from build123d import *

# Parameters (mm, degrees)
SKETCH1_R           = 20
BOSS_EXTRUDE1_DEPTH = 7
SKETCH2_R           = 8.5
CUT_EXTRUDE1_DEPTH  = 5
SKETCH3_R           = 4.5
CUT_EXTRUDE2_DEPTH  = 29.722813233
SKETCH4_R           = 1
CUT_EXTRUDE3_DEPTH  = 5
FILLET1_R           = 1


with BuildPart() as part:
    # Sketch1 → Boss-Extrude1 (new body)
    with BuildSketch(Plane(origin=(0, 0, 0), x_dir=(1, 0, 0), z_dir=(0, 1, 0))):
        with Locations(Location((0, 0, 0), (0, 0, 270))):
            Circle(SKETCH1_R)
    extrude(amount=BOSS_EXTRUDE1_DEPTH)

    # Sketch2 → Cut-Extrude1 (cut)
    with BuildSketch(Plane(origin=(0, 7, 0), x_dir=(1, 0, 0), z_dir=(0, 1, 0))):
        with Locations(Location((0, 0, 0), (0, 0, 270))):
            Circle(SKETCH2_R)
    extrude(amount=-CUT_EXTRUDE1_DEPTH, mode=Mode.SUBTRACT)

    # Sketch3 → Cut-Extrude2 (cut, through all)
    with BuildSketch(Plane(origin=(0, 2, 0), x_dir=(1, 0, 0), z_dir=(0, 1, 0))):
        with Locations(Location((0, 0, 0), (0, 0, 270))):
            Circle(SKETCH3_R)
    extrude(amount=-CUT_EXTRUDE2_DEPTH, mode=Mode.SUBTRACT)

    # Sketch4 → Cut-Extrude3 (cut)
    with BuildSketch(Plane(origin=(0, 7, 0), x_dir=(1, 0, 0), z_dir=(0, 1, 0))):
        with Locations(Location((0, 18, 0), (0, 0, 270))):
            Circle(SKETCH4_R)
        with Locations(Location((9, 15.588457268, 0), (0, 0, 270))):
            Circle(SKETCH4_R)
        with Locations(Location((15.588457268, 9, 0), (0, 0, 270))):
            Circle(SKETCH4_R)
        with Locations(Location((18, 0, 0), (0, 0, 270))):
            Circle(SKETCH4_R)
        with Locations(Location((15.588457268, -9, 0), (0, 0, 270))):
            Circle(SKETCH4_R)
        with Locations(Location((9, -15.588457268, 0), (0, 0, 270))):
            Circle(SKETCH4_R)
        with Locations(Location((0, -18, 0), (0, 0, 270))):
            Circle(SKETCH4_R)
        with Locations(Location((-9, -15.588457268, 0), (0, 0, 270))):
            Circle(SKETCH4_R)
        with Locations(Location((-15.588457268, -9, 0), (0, 0, 270))):
            Circle(SKETCH4_R)
        with Locations(Location((-18, 0, 0), (0, 0, 270))):
            Circle(SKETCH4_R)
        with Locations(Location((-15.588457268, 9, 0), (0, 0, 270))):
            Circle(SKETCH4_R)
        with Locations(Location((-9, 15.588457268, 0), (0, 0, 270))):
            Circle(SKETCH4_R)
    extrude(amount=-CUT_EXTRUDE3_DEPTH, mode=Mode.SUBTRACT)

    # Fillet1
    fillet1_edges = [part.edges().sort_by_distance(p)[0] for p in [
        (0, 0, -20),
    ]]
    fillet(fillet1_edges, radius=FILLET1_R)


solid = part.part
CAD build for the part. Positions are in the model's coordinates, mm. A direction names the side the tool comes from. Round coordinates to 2 decimals unless told otherwise and drop trailing zeros. Order: outer loops, then holes, each group sorted by start corner. A loop starts at its lowest first (then second) coordinate and runs counter-clockwise, first axis right, second up. Notation, with made-up numbers: M -30,-3.75 L -11,-3.75 A27 cw -11,35.25 Z; hole C 17,-30.75 d5. An arc over 180 degrees is marked long. Use one line per item in the form item = value.
Q1. Saw through at A-A on z = 0. Give the cut face in (x, y), then the cut area to 3 significant figures.
Recorded:
outline = M -20,1 A1 ccw -19,0 L -4.5,0 L -4.5,2 L -8.5,2 L -8.5,7 L -17,7 L -17,2 L -19,2 L -19,7 L -20,7 Z; M 4.5,0 L 19,0 A1 ccw 20,1 L 20,7 L 19,7 L 19,2 L 17,2 L 17,7 L 8.5,7 L 8.5,2 L 4.5,2 Z
area = 157 mm^2
Q2. Probe L1, parallel to X at y = 5.4, z = 0; L2, parallel to X at y = 6, z = 15; L3, parallel to X at y = 3.85, z = 9. List the from-to ranges inside material, lowest first.
Recorded:
L1 = -20 to -19, -17 to -8.5, 8.5 to 17, 19 to 20
L2 = -13.23 to -9.81, -8.19 to 8.19, 9.81 to 13.23
L3 = -17.86 to -16.59, -14.59 to 14.59, 16.59 to 17.86
Q3. Saw through at B-B on x = 0. Give the cut face in (y, z), then the cut area to 3 significant figures.
Recorded:
outline = M 0,-19 A1 ccw 1,-20 L 7,-20 L 7,-19 L 2,-19 L 2,-17 L 7,-17 L 7,-8.5 L 2,-8.5 L 2,-4.5 L 0,-4.5 Z; M 0,4.5 L 2,4.5 L 2,8.5 L 7,8.5 L 7,17 L 2,17 L 2,19 L 7,19 L 7,20 L 1,20 A1 ccw 0,19 Z
area = 157 mm^2
Q4. Flat gauge pins, fed straight in: P1, Ø4, axis at y = 2, z = 14, coming from the -X side; P2, Ø1, axis at x = 16, z = -9, coming from the +Y side; P3, Ø2, axis at x = 3.5, y = 3.5, coming from the -Z side. Where does each tip first touch, or does it go through?
Recorded:
P1 = -16
P2 = 2
P3 = -19.84
Q5. Two-plate mould, pull along X, no slides. Class faces 1 (the flat face through (0, 7, 9)), 2 (the cylindrical face through (-19.524, 3.958, -4.336)), 3 (the cylindrical face through (8.428, 4.535, -1.107)): +X half, -X half, draft (parallel to the pull), parting line (faces both ways), or undercut.
Recorded:
face_1 = draft
face_2 = parting line
face_3 = undercut
Q6. Which spindle directions (+Z, -Z, +X, -X, +Y, -Y) get a long thin tool onto all of the face, cutting with end or side? Do faces 4 (the cylindrical face through (9.99, 4.54, 15.46)), 5 (the flat face through (-4, 0, 4)). Say none if no direction does.
Recorded:
face_4 = +Y
face_5 = +Z, -Z, +X, -X, -Y
